from build123d import *

# Parameters (mm, degrees)
SKETCH1_R           = 17.5
SKETCH1_R_2         = 2.5
SKETCH1_R_3         = 6
BOSS_EXTRUDE1_DEPTH = 5


with BuildPart() as part:
    # Sketch1 → Boss-Extrude1 (new body)
    with BuildSketch(Plane.XY):
        Polygon((80, 55.80696734), (-80, 55.80696734), (-105, 41.595146974), (-105, -43.404853026), (-80.384405058, -57.616673392), (80.384405058, -57.616673392), (105, -43.404853026), (105, 41.595146974), align=None)
        with Locations((0, -0.904853026)):
            Circle(SKETCH1_R, mode=Mode.SUBTRACT)
        with Locations((-95, 14.095146974)):
            Circle(SKETCH1_R_2, mode=Mode.SUBTRACT)
        with Locations((-80, 14.095146974)):
            Circle(SKETCH1_R_2, mode=Mode.SUBTRACT)
        with Locations((-95, -15.904853026)):
            Circle(SKETCH1_R_2, mode=Mode.SUBTRACT)
        with Locations((-80, -15.904853026)):
            Circle(SKETCH1_R_2, mode=Mode.SUBTRACT)
        with Locations(Location((80, -15.904853026, 0), (0, 0, 180))):
            Circle(SKETCH1_R_2, mode=Mode.SUBTRACT)
        with Locations(Location((95, -15.904853026, 0), (0, 0, 180))):
            Circle(SKETCH1_R_2, mode=Mode.SUBTRACT)
        with Locations(Location((95, 14.095146974, 0), (0, 0, 180))):
            Circle(SKETCH1_R_2, mode=Mode.SUBTRACT)
        with Locations(Location((80, 14.095146974, 0), (0, 0, 180))):
            Circle(SKETCH1_R_2, mode=Mode.SUBTRACT)
        with Locations((-41.5, 40.595146974)):
            Circle(SKETCH1_R_3, mode=Mode.SUBTRACT)
        with Locations((41.5, 40.595146974)):
            Circle(SKETCH1_R_3, mode=Mode.SUBTRACT)
        with Locations((41.5, -42.404853026)):
            Circle(SKETCH1_R_3, mode=Mode.SUBTRACT)
        with Locations((-41.5, -42.404853026)):
            Circle(SKETCH1_R_3, mode=Mode.SUBTRACT)
    extrude(amount=BOSS_EXTRUDE1_DEPTH)


solid = part.part
Geometry check sheet. Reference: the model listing, model coordinates, mm. Coordinates: 2 decimals unless noted, no trailing zeros. Loops run counter-clockwise (first coordinate to the right, second up) from the corner with the lowest first, then second, coordinate; pieces in that order, holes last. Notation, with made-up numbers: (-10, -19.5) - (28, -19.5) arc R22 ccw to (28, 14.5) - close; hole circle Ø8 at (-23.75, 69). An arc over 180 degrees is marked (long way). Use one line per item in the form item = value. Start each with the question number.
Item 1: Section check B-B, the plane x = 0. Enter the section's corners in (y, z).
Item 2: Section check D-D, the plane x = 95. Enter the section's corners in (y, z), and give its area (3 significant figures).
Item 3: Thickness scan on probe 1 along Y at (x, z) = (80, 2.05); probe 2 along Y at (x, z) = (41.5, 3.2); probe 3 along X at (y, z) = (39.5, 0.4). Record the ranges inside material, lowest first.
Item 4: Gauge pin test, flat ends, axial feed: pin 1 (9.5 mm diameter, centred on x = 41.5, y = 40.6, fed in from +Z); pin 2 (15.5 mm diameter, centred on x = 41.5, y = -42.4, fed in from +Z). Record the tip position at first contact, or that the pin passes through.
Item 5: Section check C-C, the plane y = -5.5. Enter the section's corners in (x, z), and give its area (3 significant figures).
Item 6: Section check A-A, the plane x = -41.5. Enter the section's corners in (y, z), and give its area (3 significant figures).
Item 7: Mould release check, pull along Y, two halves, no side actions. Record for faces 1 (the face through (92.52, -50.61, 2.46)), 2 (the face through (22, 0, 0)), 3 (the face through (96.98, -14.38, 2.46)), 4 (the face through (92.68, 48.6, 2.46)): +Y half, -Y half, draft (parallel to the pull), parting line (faces both ways), or undercut.
Computed:
q1.outline = (-57.62, 0) - (-18.4, 0) - (-18.4, 5) - (-57.62, 5) - close; (16.6, 0) - (55.81, 0) - (55.81, 5) - (16.6, 5) - close
q2.outline = (-49.18, 0) - (-18.4, 0) - (-18.4, 5) - (-49.18, 5) - close; (-13.4, 0) - (11.6, 0) - (11.6, 5) - (-13.4, 5) - close; (16.6, 0) - (47.28, 0) - (47.28, 5) - (16.6, 5) - close
q2.area = 432 mm2
q3.probe_1 = -57.62 to -18.4, -13.4 to 11.6, 16.6 to 55.81
q3.probe_2 = -57.62 to -48.4, -36.4 to 34.6, 46.6 to 55.81
q3.probe_3 = -105 to -47.4, -35.6 to 35.6, 47.4 to 105
q4.pin_1 = through
q4.pin_2 = 5
q5.outline = (-105, 0) - (-16.89, 0) - (-16.89, 5) - (-105, 5) - close; (16.89, 0) - (105, 0) - (105, 5) - (16.89, 5) - close
q5.area = 881 mm2
q6.outline = (-57.62, 0) - (-48.4, 0) - (-48.4, 5) - (-57.62, 5) - close; (-36.4, 0) - (34.6, 0) - (34.6, 5) - (-36.4, 5) - close; (46.6, 0) - (55.81, 0) - (55.81, 5) - (46.6, 5) - close
q6.area = 447 mm2
q7.face_1 = -Y half
q7.face_2 = draft
q7.face_3 = undercut
q7.face_4 = +Y half
